from build123d import *

# Parameters (mm, degrees)
SKETCH1_W           = 59
SKETCH1_H           = 44
SKETCH1_R           = 1.75
BOSS_EXTRUDE1_DEPTH = 7.5
BOSS_EXTRUDE2_DEPTH = 59


with BuildPart() as part:
    # Sketch1 → Boss-Extrude1 (new body)
    with BuildSketch(Plane(origin=(0, 0, 0), x_dir=(1, 0, 0), z_dir=(0, 1, 0))):
        with Locations((29.5, 22)):
            Rectangle(SKETCH1_W, SKETCH1_H)
        with Locations(Location((15, 10.5, 0), (0, 0, 270))):
            Circle(SKETCH1_R, mode=Mode.SUBTRACT)
        with Locations(Location((44, 10.5, 0), (0, 0, 90))):
            Circle(SKETCH1_R, mode=Mode.SUBTRACT)
        with Locations(Location((15, 33.5, 0), (0, 0, 90))):
            Circle(SKETCH1_R, mode=Mode.SUBTRACT)
        with Locations(Location((44, 33.5, 0), (0, 0, 270))):
            Circle(SKETCH1_R, mode=Mode.SUBTRACT)
    extrude(amount=BOSS_EXTRUDE1_DEPTH)

    # Sketch3 → Boss-Extrude2 (add)
    with BuildSketch(Plane(origin=(59, 0, 0), x_dir=(0, 0, -1), z_dir=(1, 0, 0))):
        Polygon((0, 7.5), (-6, 10.964101615), (-6, -3.464101615), (0, 0), align=None)
        Polygon((44, 7.5), (50, 10.964101615), (50, -3.464101615), (44, 0), align=None)
    extrude(amount=-BOSS_EXTRUDE2_DEPTH)


solid = part.part
Design review of the part built by this model. Coordinates are the model's own, in mm. A direction names the side the tool comes from. Coordinates: 2 decimals unless noted, no trailing zeros. Loops run counter-clockwise (first coordinate to the right, second up) from the corner with the lowest first, then second, coordinate; pieces in that order, holes last. Notation, with made-up numbers: M 15.25,-34.5 L 51.25,-34.5 A23 cw 51.25,-1.5 Z; hole C -16.5,-11.5 d1. An arc over 180 degrees is marked long. Answer as CSV lines item,"result".
Item 1: For probe 1 along X at (y, z) = (6, -33.5); probe 2 along X at (y, z) = (4.25, -32); probe 3 along Z at (x, y) = (44.5, 5.5), list the stretches that pass through material, from the lowest coordinate up.
Answer list:
probe 1,"0 to 13.25, 16.75 to 42.25, 45.75 to 59"
probe 2,"0 to 14.1, 15.9 to 43.1, 44.9 to 59"
probe 3,"-50 to -35.18, -31.82 to -12.18, -8.82 to 6"
Item 2: For P1, Ø4, axis at x = 36, z = -21.5, coming from the -Y side; P2, Ø22, axis at x = 22, z = -19.5, coming from the +Y side, all flat-tipped, find the tip position at first contact; note any pin that passes through.
Answer list:
P1,"y = 0"
P2,"y = 7.5"
Item 3: Add section D-D on y = -1.75. State the section outline as (x, z) points.
Answer list:
outline,"M 0,-50 L 59,-50 L 59,-47.03 L 0,-47.03 Z; M 0,3.03 L 59,3.03 L 59,6 L 0,6 Z"
Item 4: Add section B-B on y = 10. State the section outline as (x, z) points.
Answer list:
outline,"M 0,-50 L 59,-50 L 59,-48.33 L 0,-48.33 Z; M 0,4.33 L 59,4.33 L 59,6 L 0,6 Z"
Item 5: Add section C-C on x = 55.5. State the section outline as (y, z) points.
Answer list:
outline,"M -3.46,-50 L 10.96,-50 L 7.5,-44 L 7.5,0 L 10.96,6 L -3.46,6 L 0,0 L 0,-44 Z"
Item 6: Machinability: for faces 1 (the face through (29, 0, -22)), 2 (the face through (16.735, 3.698, -10.728)), 3 (the face through (29, 7.5, -22)), which of the approach directions +Z, -Z, +X, -X, +Y, -Y give a long, thin tool a straight path to every point of the face, cutting with its end or side? Answer none if there is none.
Answer list:
face 1,"+X, -X, -Y"
face 2,"+Y, -Y"
face 3,"+X, -X, +Y"
Item 7: Add section A-A on x = 44. State the section outline as (y, z) points, plus the area to 3 significant figures.
Answer list:
outline,"M -3.46,-50 L 10.96,-50 L 7.5,-44 L 7.5,-35.25 L 0,-35.25 L 0,-44 Z; M -3.46,6 L 0,0 L 0,-8.75 L 7.5,-8.75 L 7.5,0 L 10.96,6 Z; M 0,-31.75 L 7.5,-31.75 L 7.5,-12.25 L 0,-12.25 Z"
area,"409 mm²"
Item 8: The part is to be moulded in two halves that separate along Z. For faces 4 (the face through (59, 4, -22)), 5 (the face through (45.71, 3.7, -10.12)), 6 (the face through (30, 4, -50)), 7 (the face through (42.29, 3.7, -33.88)), say which applies: pulls with the +Z half, pulls with the -Z half, needs draft (parallel to the pull), parting line crosses it, or undercut.
Answer list:
face 4,"needs draft"
face 5,"undercut"
face 6,"pulls with the -Z half"
face 7,"undercut"
